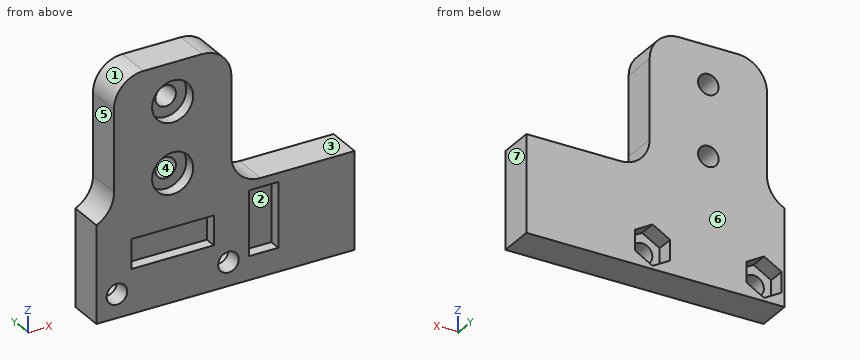
from build123d import *

# Parameters (mm, degrees)
F0_R        = 1.75
F0_W        = 14
F0_H        = 5
F0_W_2      = 5
F0_H_2      = 11
F0_R_2      = 3.5
F1_DEPTH    = 6
F2_DEPTH    = 2
F4_DEPTH    = 3
F5_T1_DEPTH = 6
F5_T3_DEPTH = 6
F5_T5_DEPTH = 31
F5_T7_DEPTH = 31


# Not quite as in the source:
# - a fillet or chamfer that OpenCascade refuses, or shapes differently, is made with other operations: its cross-section is extruded or revolved along the edge and cut away or added


with BuildPart() as f1:
    # F0 (on Front) → F1 (new body)
    with BuildSketch(Plane.XZ):
        Polygon((-11.5, -20), (32.5, -20), (32.5, -3.5), (11.5, -3.5), (11.5, 20), (-8.5, 20), (-8.5, -3.5), (-11.5, -3.5), align=None)
        with Locations((-8, -16)):
            Circle(F0_R, mode=Mode.SUBTRACT)
        with Locations((1.5, -10)):
            Rectangle(F0_W, F0_H, mode=Mode.SUBTRACT)
        with Locations((11, -16)):
            Circle(F0_R, mode=Mode.SUBTRACT)
        with Locations((17, -10.5)):
            Rectangle(F0_W_2, F0_H_2, mode=Mode.SUBTRACT)
        with Locations((1.5, 1.5)):
            Circle(F0_R_2, mode=Mode.SUBTRACT)
        with Locations((1.5, 13.5)):
            Circle(F0_R_2, mode=Mode.SUBTRACT)
        with Locations((1.5, -10)):
            Rectangle(F0_W, F0_H)
        with Locations((17, -10.5)):
            Rectangle(F0_W_2, F0_H_2)
        with Locations((1.5, 1.5)):
            Circle(F0_R_2)
        with Locations((1.5, 1.5)):
            Circle(F0_R, mode=Mode.SUBTRACT)
        with Locations((1.5, 13.5)):
            Circle(F0_R_2)
        with Locations((1.5, 13.5)):
            Circle(F0_R, mode=Mode.SUBTRACT)
    extrude(amount=-F1_DEPTH)

    # F0 (on Front) → F2 (cut)
    with BuildSketch(Plane.XZ):
        with Locations((17, -10.5)):
            Rectangle(F0_W_2, F0_H_2)
        with Locations((1.5, -10)):
            Rectangle(F0_W, F0_H)
        with Locations((1.5, 13.5)):
            Circle(F0_R_2)
        with Locations((1.5, 13.5)):
            Circle(F0_R, mode=Mode.SUBTRACT)
        with Locations((1.5, 1.5)):
            Circle(F0_R_2)
        with Locations((1.5, 1.5)):
            Circle(F0_R, mode=Mode.SUBTRACT)
    extrude(amount=-F2_DEPTH, mode=Mode.SUBTRACT)

    # F3 (on face) → F4 (cut)
    with BuildSketch(Plane(origin=(0, 6, 0), x_dir=(-1, 0, 0), z_dir=(0, 1, 0))):
        Polygon((-11, -12.5358983849), (-14, -14.2679491924), (-14, -17.7320508076), (-11, -19.4641016151), (-8, -17.7320508076), (-8, -14.2679491924), align=None)
        Polygon((5, -14.2679491924), (5, -17.7320508076), (8, -19.4641016151), (11, -17.7320508076), (11, -14.2679491924), (8, -12.5358983849), align=None)
    extrude(amount=-F4_DEPTH, mode=Mode.SUBTRACT)

    # F5: fillet of radius 5 on 4 edges, made by hand

    # F5_s2 → F5_t1 (join)
    with BuildSketch(Plane.XZ.offset(-6)):
        with BuildLine():
            ThreePointArc((-11.5, -3.5), (-9.3166998673, -1.6560370926), (-8.5, 1.082575695))
            Line((-8.5, 1.082575695), (-8.5, -3.5))
            Line((-8.5, -3.5), (-11.5, -3.5))
        make_face()
    extrude(amount=F5_T1_DEPTH)

    # F5_s4 → F5_t3 (join)
    with BuildSketch(Plane.XZ.offset(-6)):
        with BuildLine():
            ThreePointArc((16.5, -3.5), (12.9644660941, -2.0355339059), (11.5, 1.5))
            Line((11.5, 1.5), (11.5, -3.5))
            Line((11.5, -3.5), (16.5, -3.5))
        make_face()
    extrude(amount=F5_T3_DEPTH)

    # F5_s6 → F5_t5 (cut)
    with BuildSketch(Plane.XZ.offset(-18.5)):
        with BuildLine():
            ThreePointArc((-3.5, 20), (-7.0355339059, 18.5355339059), (-8.5, 15))
            Line((-8.5, 15), (-8.5, 20))
            Line((-8.5, 20), (-3.5, 20))
        make_face()
    extrude(amount=F5_T5_DEPTH, mode=Mode.SUBTRACT)

    # F5_s8 → F5_t7 (cut)
    with BuildSketch(Plane.XZ.offset(-18.5)):
        with BuildLine():
            ThreePointArc((6.5, 20), (10.0355339059, 18.5355339059), (11.5, 15))
            Line((11.5, 15), (11.5, 20))
            Line((11.5, 20), (6.5, 20))
        make_face()
    extrude(amount=F5_T7_DEPTH, mode=Mode.SUBTRACT)


solid = f1.part
For this review, take the finished solid that the model builds, in its own axes (mm). Face numbers are marked on the shaded views. A direction names the side the tool comes from. Coordinates: 2 decimals unless noted, no trailing zeros. Order: outer loops, then holes, each group sorted by start corner. A loop starts at its lowest first (then second) coordinate and runs counter-clockwise, first axis right, second up. Notation, with made-up numbers: (40.25, 87) - (45.25, 87) arc R15 cw to (45.25, 108) - close; hole circle Ø4 at (70.5, 78). An arc over 180 degrees is marked (long way). Use one line per item in the form item = value.
Q1. For the marked faces 1, 2 and 3, list the 3-axis set-ups (+Z, -Z, +X, -X, +Y, -Y) from which the entire face can be reached by the end or side of a thin tool; tool diameter is ignored.
Checked values:
face_1 = +Z, -X, +Y, -Y
face_2 = -Y
face_3 = +Z, +X, +Y, -Y
Q2. Consider section A-A (x = 1.5). Give the boundary of the cut face in (y, z), then the cut area to 3 significant figures.
Checked values:
outline = (0, -20) - (6, -20) - (6, -0.25) - (2, -0.25) - (2, -2) - (0, -2) - (0, -7.5) - (2, -7.5) - (2, -12.5) - (0, -12.5) - close; (0, 5) - (2, 5) - (2, 3.25) - (6, 3.25) - (6, 11.75) - (2, 11.75) - (2, 10) - (0, 10) - close; (0, 17) - (2, 17) - (2, 15.25) - (6, 15.25) - (6, 20) - (0, 20) - close
area = 174 mm2
Q3. Consider section C-C (z = -11.5). Give the boundary of the cut face in (x, y).
Checked values:
outline = (-11.5, 0) - (-5.5, 0) - (-5.5, 2) - (8.5, 2) - (8.5, 0) - (14.5, 0) - (14.5, 2) - (19.5, 2) - (19.5, 0) - (32.5, 0) - (32.5, 6) - (-11.5, 6) - close
Q4. Consider section B-B (y = 5.5). Give the boundary of the cut face in (x, z), then the cut area to 3 significant figures.
Checked values:
outline = (-11.5, -20) - (32.5, -20) - (32.5, -3.5) - (16.5, -3.5) arc R5 cw to (11.5, 1.5) - (11.5, 15) arc R5 ccw to (6.5, 20) - (-3.5, 20) arc R5 ccw to (-8.5, 15) - (-8.5, 1.08) arc R5 cw to (-11.5, -3.5) - close; hole (-11, -17.73) - (-8, -19.46) - (-5, -17.73) - (-5, -14.27) - (-8, -12.54) - (-11, -14.27) - close; hole circle Ø3.5 at (1.5, 1.5); hole circle Ø3.5 at (1.5, 13.5); hole (8, -17.73) - (11, -19.46) - (14, -17.73) - (14, -14.27) - (11, -12.54) - (8, -14.27) - close
area = 1,110 mm2
Q5. For P1, Ø2, axis at x = 17, y = 1, coming from the +Z side; P2, Ø1, axis at y = 2.5, z = 10.5, coming from the -X side; P3, Ø5.5, axis at x = 1.5, z = 13.5, coming from the -Y side, all flat-tipped, find the tip position at first contact; note any pin that passes through.
Checked values:
P1 = -3.47
P2 = -8.5
P3 = 2
Q6. Consider section D-D (x = 26.5). Give the boundary of the cut face in (y, z).
Checked values:
outline = (0, -20) - (6, -20) - (6, -3.5) - (0, -3.5) - close
Q7. Draft analysis for pull direction X (two halves, no side actions). For the marked faces 4, 5, 6 and 7, state which applies: +X half, -X half, draft (parallel to the pull), parting line (faces both ways), or undercut.
Checked values:
face_4 = undercut
face_5 = -X half
face_6 = draft
face_7 = +X half
Q8. For probe 1 along X at (y, z) = (5.2, -15); probe 2 along Z at (x, y) = (1.5, 3.3); probe 3 along Z at (x, y) = (1.5, 1.6), list the stretches that pass through material, from the lowest coordinate up. Write a range as from..to.
Checked values:
probe_1 = -11.5..-11, -5..8, 14..32.5
probe_2 = -20..-0.25, 3.25..11.75, 15.25..20
probe_3 = -20..-12.5, -7.5..-2, 5..10, 17..20
